```python
from build123d import *

# Parameters (mm, degrees)
SKETCH1_W           = 88
SKETCH1_H           = 46
SKETCH1_W_2         = 82
SKETCH1_H_2         = 40
BOSS_EXTRUDE1_DEPTH = 3
SKETCH3_W           = 88
SKETCH3_H           = 46
BOSS_EXTRUDE2_DEPTH = 200
SKETCH6_W           = 10
SKETCH6_H           = 10
SKETCH6_R           = 2.5
BOSS_EXTRUDE4_DEPTH = 10


with BuildPart() as part:
    # Sketch1 → Boss-Extrude1 (new body)
    # profile 1 of 2: a face of its own
    with BuildSketch(Plane.XY):
        with Locations((-44, -23)):
            Rectangle(SKETCH1_W, SKETCH1_H)
        with Locations((-44, -23)):
            Rectangle(SKETCH1_W_2, SKETCH1_H_2, mode=Mode.SUBTRACT)
    # profile 2 of 2: a face of its own
    with BuildSketch(Plane.XY):
        with Locations((-44, -23)):
            Rectangle(SKETCH1_W_2, SKETCH1_H_2)
    extrude(amount=BOSS_EXTRUDE1_DEPTH)

    # Sketch3 → Boss-Extrude2 (add)
    with BuildSketch(Plane(origin=(0, 0, 0), x_dir=(-1, 0, 0), z_dir=(0, 0, -1))):
        with Locations((44, -23)):
            Rectangle(SKETCH3_W, SKETCH3_H)
        Polygon((24, -3), (43, -3), (43, -1.5), (45, -1.5), (45, -3), (64, -3), (64, -1.5), (66, -1.5), (66, -3), (85, -3), (85, -43), (66, -43), (66, -44.5), (64, -44.5), (64, -43), (45, -43), (45, -44.5), (43, -44.5), (43, -43), (24, -43), (24, -44.5), (22, -44.5), (22, -43), (3, -43), (3, -3), (22, -3), (22, -1.5), (24, -1.5), align=None, mode=Mode.SUBTRACT)
    extrude(amount=BOSS_EXTRUDE2_DEPTH)

    # Sketch6 → Boss-Extrude4 (add)
    # profile 1 of 10: a face of its own
    with BuildSketch(Plane(origin=(0, 0, 0), x_dir=(1, 0, 0), z_dir=(0, 1, 0))):
        with Locations((-93, 98.5)):
            Rectangle(SKETCH6_W, SKETCH6_H)
        with Locations(Location((-93, 98.5, 0), (0, 0, 270))):
            Circle(SKETCH6_R, mode=Mode.SUBTRACT)
    # profile 2 of 10: a face of its own
    with BuildSketch(Plane(origin=(0, 0, 0), x_dir=(1, 0, 0), z_dir=(0, 1, 0))):
        with Locations((5, 98.5)):
            Rectangle(SKETCH6_W, SKETCH6_H)
        with Locations(Location((5, 98.5, 0), (0, 0, 270))):
            Circle(SKETCH6_R, mode=Mode.SUBTRACT)
    # profile 3 of 10: a face of its own
    with BuildSketch(Plane(origin=(0, 0, 0), x_dir=(1, 0, 0), z_dir=(0, 1, 0))):
        with Locations((-93, 137.5)):
            Rectangle(SKETCH6_W, SKETCH6_H)
        with Locations(Location((-93, 137.5, 0), (0, 0, 270))):
            Circle(SKETCH6_R, mode=Mode.SUBTRACT)
    # profile 4 of 10: a face of its own
    with BuildSketch(Plane(origin=(0, 0, 0), x_dir=(1, 0, 0), z_dir=(0, 1, 0))):
        with Locations((5, 137.5)):
            Rectangle(SKETCH6_W, SKETCH6_H)
        with Locations(Location((5, 137.5, 0), (0, 0, 270))):
            Circle(SKETCH6_R, mode=Mode.SUBTRACT)
    # profile 5 of 10: a face of its own
    with BuildSketch(Plane(origin=(0, 0, 0), x_dir=(1, 0, 0), z_dir=(0, 1, 0))):
        with Locations((-93, 59.5)):
            Rectangle(SKETCH6_W, SKETCH6_H)
        with Locations(Location((-93, 59.5, 0), (0, 0, 270))):
            Circle(SKETCH6_R, mode=Mode.SUBTRACT)
    # profile 6 of 10: a face of its own
    with BuildSketch(Plane(origin=(0, 0, 0), x_dir=(1, 0, 0), z_dir=(0, 1, 0))):
        with Locations((5, 59.5)):
            Rectangle(SKETCH6_W, SKETCH6_H)
        with Locations(Location((5, 59.5, 0), (0, 0, 270))):
            Circle(SKETCH6_R, mode=Mode.SUBTRACT)
    # profile 7 of 10: a face of its own
    with BuildSketch(Plane(origin=(0, 0, 0), x_dir=(1, 0, 0), z_dir=(0, 1, 0))):
        with Locations((-93, 13)):
            Rectangle(SKETCH6_W, SKETCH6_H)
        with Locations(Location((-93, 13, 0), (0, 0, 270))):
            Circle(SKETCH6_R, mode=Mode.SUBTRACT)
    # profile 8 of 10: a face of its own
    with BuildSketch(Plane(origin=(0, 0, 0), x_dir=(1, 0, 0), z_dir=(0, 1, 0))):
        with Locations((5, 13)):
            Rectangle(SKETCH6_W, SKETCH6_H)
        with Locations(Location((5, 13, 0), (0, 0, 270))):
            Circle(SKETCH6_R, mode=Mode.SUBTRACT)
    # profile 9 of 10: a face of its own
    with BuildSketch(Plane(origin=(0, 0, 0), x_dir=(1, 0, 0), z_dir=(0, 1, 0))):
        with Locations((5, 184)):
            Rectangle(SKETCH6_W, SKETCH6_H)
        with Locations(Location((5, 184, 0), (0, 0, 270))):
            Circle(SKETCH6_R, mode=Mode.SUBTRACT)
    # profile 10 of 10: a face of its own
    with BuildSketch(Plane(origin=(0, 0, 0), x_dir=(1, 0, 0), z_dir=(0, 1, 0))):
        with Locations((-93, 184)):
            Rectangle(SKETCH6_W, SKETCH6_H)
        with Locations(Location((-93, 184, 0), (0, 0, 270))):
            Circle(SKETCH6_R, mode=Mode.SUBTRACT)
    extrude(amount=-BOSS_EXTRUDE4_DEPTH)


solid = part.part
```
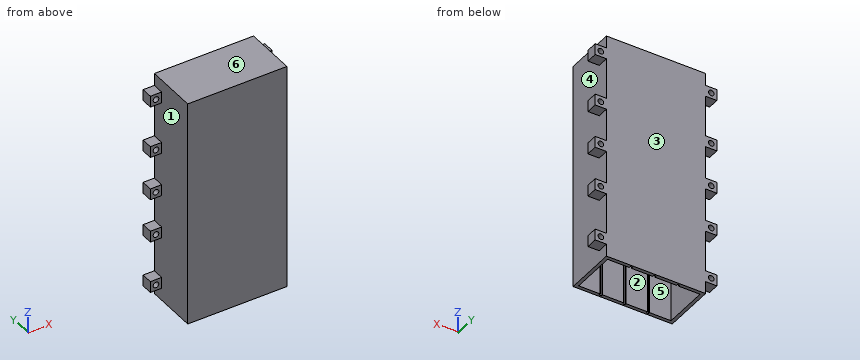
For this review, take the finished solid that the model builds, in its own axes (mm). Face numbers are marked on the shaded views. A direction names the side the tool comes from. Round coordinates to 2 decimals unless told otherwise and drop trailing zeros. Write each loop counter-clockwise with the first axis right and the second up, starting at its lowest first coordinate (ties: lowest second). Pieces come first, ordered by that corner, then holes.
1) For line 1 along X through (y, z) = (-6.5, -137.5); line 2 along Y through (x, z) = (-48, -139); line 3 along X through (y, z) = (-17, -86.5), list the stretches that pass through material, from the lowest coordinate up.
Answer below:
line 1: x = -98 to -95.5, -90.5 to -85, -3 to 2.5, 7.5 to 10
line 2: y = -46 to -43, -3 to 0
line 3: x = -88 to -85, -3 to 0
2) Take a section at D-D on z = -98.5. State how many separate pieces and enclosed holes the cut face has, then the cut area to 3 significant figures.
Answer below:
separate pieces: 3
enclosed holes: 1
area: 850 mm2
3) Insertion check: pin 1 Ø10 at (x, y) = (-48, -25) entering from -Z; pin 2 Ø5 at (y, z) = (-28.5, -34.5) entering from -X; pin 3 Ø12 at (y, z) = (-27, -140) entering from +X; pin 4 Ø3 at (x, z) = (5, -137.5) entering from +Y. Each pin has a flat end and moves straight along its axis. Give the tip position at first contact, or say it passes through.
Answer below:
pin 1: stops at z = 0
pin 2: stops at x = -88
pin 3: stops at x = 0
pin 4: passes through
4) Machinability: for the marked faces 5 and 6, which of the approach directions +Z, -Z, +X, -X, +Y, -Y give a long, thin tool a straight path to every point of the face, cutting with its end or side? Answer none if there is none.
Answer below:
face 5: -Z
face 6: +Z, +X, -X, +Y, -Y
5) Mouldability with a two-part tool opening along X and no side actions: class the marked faces 1, 2, 3 and 4 as +X half, -X half, draft (parallel to the pull), parting line (faces both ways), or undercut.
Answer below:
face 1: -X half
face 2: undercut
face 3: draft
face 4: +X half
6) Take a section at B-B on x = -30. Give the boundary of the cut face in (y, z), then the cut area to 3 significant figures.
Answer below:
outline: (-46, -200) - (-43, -200) - (-43, 0) - (-3, 0) - (-3, -200) - (0, -200) - (0, 3) - (-46, 3) - close
area: 1,340 mm2
7) Take a section at C-C on y = -29.5. Give the boundary of the cut face in (x, z), then the cut area to 3 significant figures.
Answer below:
outline: (-88, -200) - (-85, -200) - (-85, 0) - (-3, 0) - (-3, -200) - (0, -200) - (0, 3) - (-88, 3) - close
area: 1,460 mm2
